The figure shows three views and two pictorial views of one solid part (mm, origin at its lowest corner). Answer the questions. Coordinates: 2 decimals unless noted, no trailing zeros. Write each loop counter-clockwise with the first axis right and the second up, starting at its lowest first coordinate (ties: lowest second). Pieces come first, ordered by that corner, then holes. Notation, with made-up numbers: M 72.25,81 L 93.25,81 A20 cw 93.25,114 Z; hole C -37.75,1 d1. An arc over 180 degrees is marked long. Use CSV: the item, a comma, the result in double quotes.
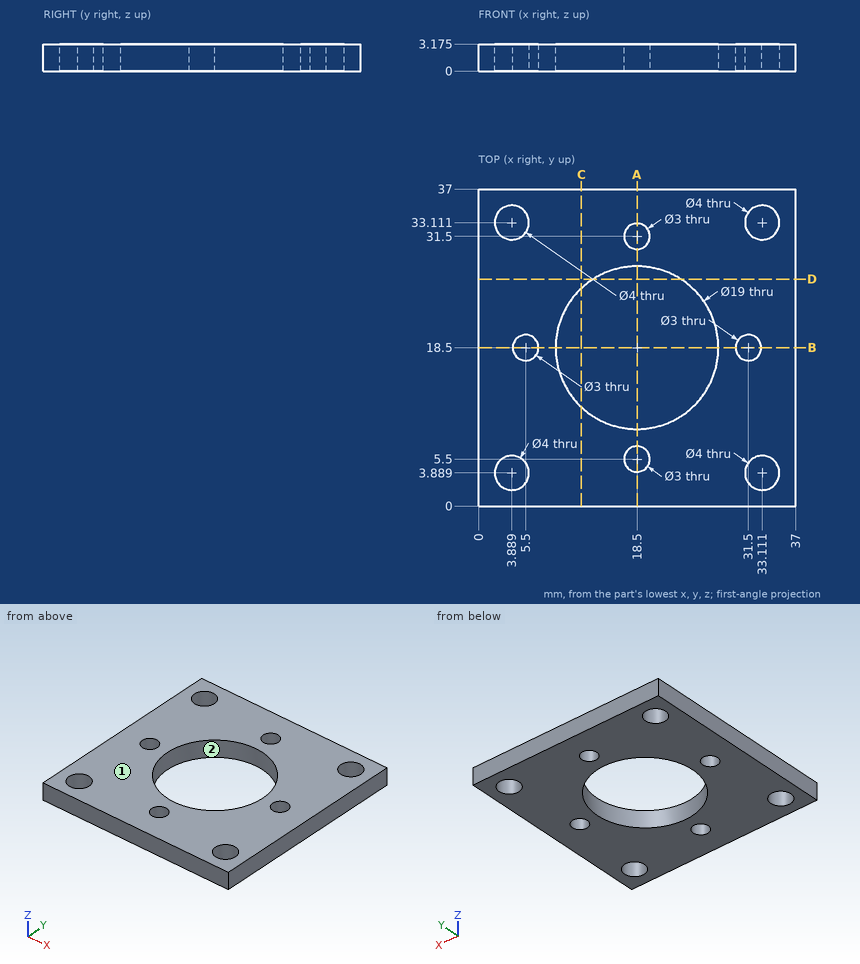
Item 1: The part is cut by section D-D (y = 26.5). Write down the section's boundary in (x, z) (1 decimal).
Answer:
outline,"M 0,0 L 13.4,0 L 13.4,3.2 L 0,3.2 Z; M 23.6,0 L 37,0 L 37,3.2 L 23.6,3.2 Z"
Item 2: Consider probe 1 along X at (y, z) = (34, 2.4); probe 2 along Y at (x, z) = (18, 0.4). Determine where each line is inside the solid, lowest interval first.
Answer:
probe 1,"x = 0 to 2.1, 5.68 to 31.32, 34.9 to 37"
probe 2,"y = 0 to 4.09, 6.91 to 9.01, 27.99 to 30.09, 32.91 to 37"
Item 3: The part is cut by section C-C (x = 12). Write down the section's boundary in (y, z) (3 decimals), then the cut area to 3 significant figures.
Answer:
outline,"M 0,0 L 11.572,0 L 11.572,3.175 L 0,3.175 Z; M 25.428,0 L 37,0 L 37,3.175 L 25.428,3.175 Z"
area,"73.5 mm2"
Item 4: The part is cut by section A-A (x = 18.5). Write down the section's boundary in (y, z) (3 decimals), then the cut area to 3 significant figures.
Answer:
outline,"M 0,0 L 4,0 L 4,3.175 L 0,3.175 Z; M 7,0 L 9,0 L 9,3.175 L 7,3.175 Z; M 28,0 L 30,0 L 30,3.175 L 28,3.175 Z; M 33,0 L 37,0 L 37,3.175 L 33,3.175 Z"
area,"38.1 mm2"
Item 5: For a pull along X with two mould halves and no side action, classify the marked faces 1 and 2 as released by +X, released by -X, zero draft, split by the parting line, or undercut.
Answer:
face 1,"zero draft"
face 2,"undercut"
Item 6: Given pin 1 (2.5 mm diameter, centred on x = 33.11, y = 33.11, fed in from +Z); pin 2 (1.5 mm diameter, centred on x = 13.5, z = 2, fed in from -Y), each flat-ended and moving along its own axis, determine where each tip first touches the part or whether it passes through.
Answer:
pin 1,"passes through"
pin 2,"stops at y = 0"
